Could you check a few things on this model? Use its own coordinates, in mm. Face numbers are marked on the shaded views. A direction names the side the tool comes from. Give positions to 0.01 mm unless a question says otherwise; leave off trailing zeros. Order: outer loops, then holes, each group sorted by start corner. A loop starts at its lowest first (then second) coordinate and runs counter-clockwise, first axis right, second up. Notation, with made-up numbers: M -12,54 L -7,54 A23 cw -7,88 Z; hole C 18,73.5 d1. An arc over 180 degrees is marked long. Use a Markdown table: item, result. Add a question column.
Item 1: If I drill on L1, parallel to X at y = -11, z = 0; L2, parallel to Y at x = 37, z = -9; L3, parallel to Y at x = -22, z = 25.5, over which ranges is the centre line in solid material (lowest first)? Write a range as from..to.
Item 2: Suppose I cut it at B-B on y = 8. Write out the boundary of the cut face in (x, z) (1 decimal), plus the area to 3 significant figures.
Item 3: Suppose I cut it at A-A on y = -2.5. Write out the boundary of the cut face in (x, z) (1 decimal), plus the area to 3 significant figures.
Item 4: For the marked faces 1 and 2, which set-ups out of +Z, -Z, +X, -X, +Y, -Y let a thin tool reach every point of the face, with its end or its side?
Item 5: I'm going to push flat-ended pins straight in: pin 1 Ø3.5 at (x, z) = (27.27, 0) entering from +Y; pin 2 Ø1.9 at (x, z) = (18.5, -32) entering from +Y; pin 3 Ø10 at (x, y) = (24, -4.5) entering from -Z. Where does each tip first touch, or does it pass through?
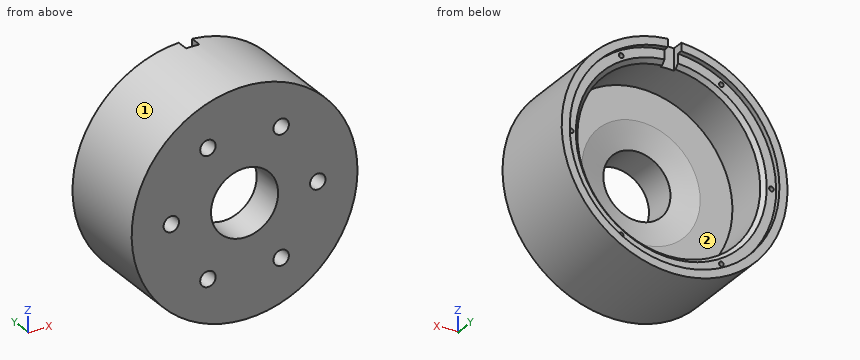
from build123d import *

# Parameters (mm, degrees)
SKETCH8_W         = 5
SKETCH8_H         = 8.09193466
WIRE_HOLE_DEPTH   = 4.5
CHAMFER1_SIZE     = 1.5
SKETCH9_R         = 0.875
FRONT_HOLES_DEPTH = 6
SKETCH10_R        = 2.875
BACK_HOLES_DEPTH  = 8


with BuildPart() as part:
    # Sketch7 → Base Motor Housing (revolve)
    with BuildSketch(Plane.XY, mode=Mode.PRIVATE) as base_motor_housing_sk:
        Polygon((-42.0375, 21.59), (-39.0375, 21.59), (-39.0375, 19.59), (-34.0375, 19.59), (-34.0375, 1.25), (-22.0375, 1.25), (-12.5, -1.25), (-12.5, -14.25), (-42.0375, -14.25), align=None)
    revolve(base_motor_housing_sk.sketch.rotate(Axis((0, -30.231871117, 0), (0, 1, 0)), 270), axis=Axis((0, -30.231871117, 0), (0, 1, 0)))

    # Sketch8 → Wire Hole (cut)
    with BuildSketch(Plane(origin=(0, 21.59, 0), x_dir=(1, 0, 0), z_dir=(0, 1, 0))):
        with Locations((0, -37.99153267)):
            Rectangle(SKETCH8_W, SKETCH8_H)
    extrude(amount=-WIRE_HOLE_DEPTH, mode=Mode.SUBTRACT)

    # Chamfer1
    chamfer1_edges = [part.edges().sort_by_distance(p)[0] for p in [
        (34.01450857, 19.59, -1.250844913),
    ]]
    chamfer(chamfer1_edges, length=CHAMFER1_SIZE)

    # Sketch9 → Front-Holes (cut)
    with BuildSketch(Plane(origin=(0, 19.59, 0), x_dir=(1, 0, 0), z_dir=(0, 1, 0))):
        with Locations(Location((-37.2875, 0, 0), (0, 0, 270))):
            Circle(SKETCH9_R)
        with Locations(Location((-18.64375, 32.291922244, 0), (0, 0, 270))):
            Circle(SKETCH9_R)
        with Locations(Location((18.64375, 32.291922244, 0), (0, 0, 270))):
            Circle(SKETCH9_R)
        with Locations(Location((37.2875, 0, 0), (0, 0, 270))):
            Circle(SKETCH9_R)
        with Locations(Location((18.64375, -32.291922244, 0), (0, 0, 270))):
            Circle(SKETCH9_R)
        with Locations(Location((-18.64375, -32.291922244, 0), (0, 0, 270))):
            Circle(SKETCH9_R)
    extrude(amount=-FRONT_HOLES_DEPTH, mode=Mode.SUBTRACT)

    # Sketch10 → Back-Holes (cut)
    with BuildSketch(Plane.XZ.offset(14.25)):
        with Locations(Location((-27.26875, 0, 0), (0, 0, 270))):
            Circle(SKETCH10_R)
        with Locations(Location((-13.634375, 23.615430229, 0), (0, 0, 270))):
            Circle(SKETCH10_R)
        with Locations(Location((13.634375, 23.615430229, 0), (0, 0, 270))):
            Circle(SKETCH10_R)
        with Locations(Location((27.26875, 0, 0), (0, 0, 270))):
            Circle(SKETCH10_R)
        with Locations(Location((13.634375, -23.615430229, 0), (0, 0, 270))):
            Circle(SKETCH10_R)
        with Locations(Location((-13.634375, -23.615430229, 0), (0, 0, 270))):
            Circle(SKETCH10_R)
    extrude(amount=-BACK_HOLES_DEPTH, mode=Mode.SUBTRACT)


solid = part.part
Findings below:
| question | item | result |
|---|---|---|
| 1 | L1 | x = -42.04..-30.14, -24.39..-12.5, 12.5..24.39, 30.14..42.04 |
| 1 | L2 | y = -14.25..19.59 |
| 1 | L3 | y = -14.25..1.25 |
| 2 | outline | C 0,0 d84.1; hole C 0,0 d68.1 |
| 2 | area | 1,910 mm^2 |
| 3 | outline | C 0,0 d84.1; hole C 0,0 d25 |
| 3 | area | 5,060 mm^2 |
| 4 | face 1 | +Y, -Y |
| 4 | face 2 | +Y |
| 5 | pin 1 | stops at y = 1.25 |
| 5 | pin 2 | stops at y = 19.59 |
| 5 | pin 3 | stops at z = -37.5 |
